The drawing under review shows one solid part. Ordinate dimensions are in mm from its lowest x, y, z. A direction names the side the tool comes from. Give positions to 0.01 mm unless a question says otherwise; leave off trailing zeros. Loops run counter-clockwise (first coordinate to the right, second up) from the corner with the lowest first, then second, coordinate; pieces in that order, holes last. Notation, with made-up numbers: (-8.75, 72) -> (22.25, 72) arc R23 cw to (22.25, 99) -> close; hole circle Ø3 at (-17.75, -3.75). An arc over 180 degrees is marked (long way). Answer in a Markdown table with one row per item. Add a question column.
(1) For pin 1 (21 mm diameter, centred on x = 19, z = 26.5, fed in from +Y); pin 2 (12 mm diameter, centred on x = 29.5, z = 24, fed in from +Y), all flat-tipped, find the tip position at first contact; note any pin that passes through.
(2) For the marked faces 1 and 2, list the 3-axis set-ups (+Z, -Z, +X, -X, +Y, -Y) from which the entire face can be reached by the end or side of a thin tool; tool diameter is ignored.
(3) Consider section C-C on y = 57.5. Write out the cut boundary in (x, z).
(4) Consider section B-B on x = 21. Write out the cut boundary in (y, z).
(5) Consider section D-D on x = 33. Write out the cut boundary in (y, z), then the cut area to 3 significant figures.
(6) Consider section A-A on z = 21. Write out the cut boundary in (x, y), then the cut area to 3 significant figures.
(7) For line 1 (Y direction, x = 12, z = 33); line 2 (X direction, y = 48, z = 22.5), list the stretches that pass through material, from the lowest coordinate up.
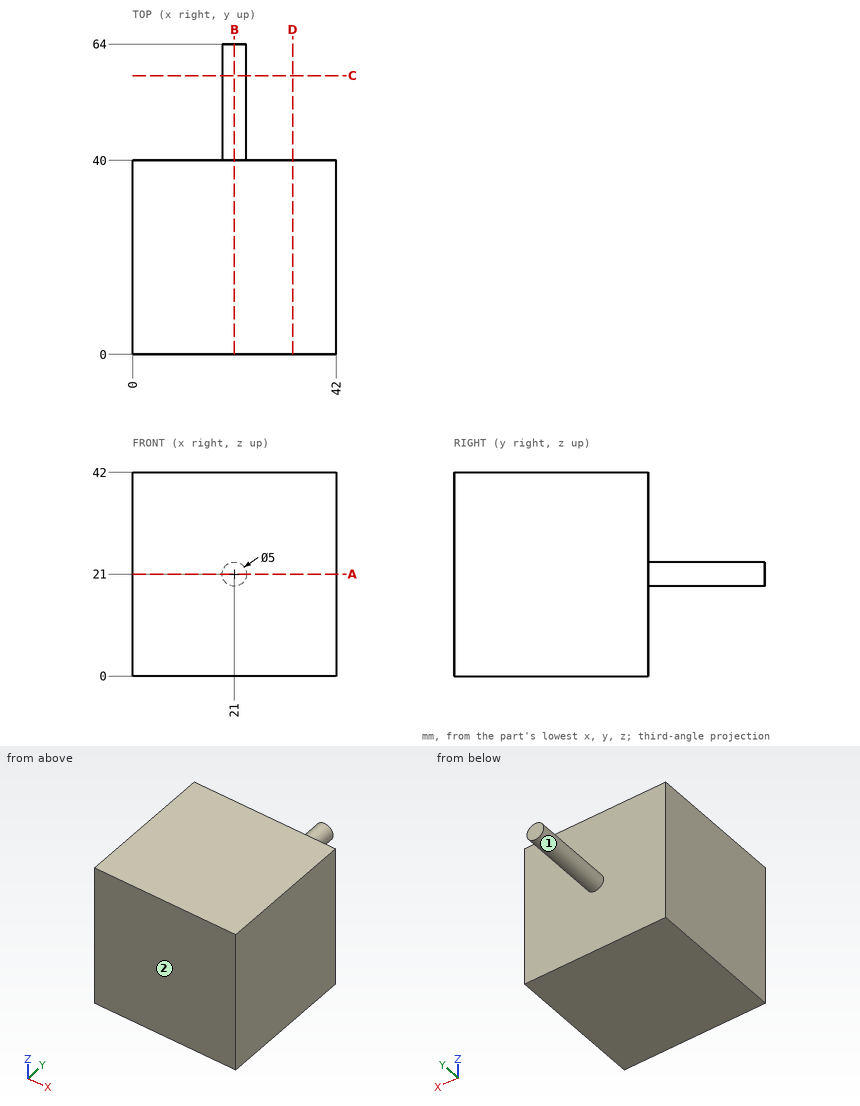
Values follow:
| question | item | result |
|---|---|---|
| 1 | pin 1 | y = 64 |
| 1 | pin 2 | y = 40 |
| 2 | face 1 | +Y |
| 2 | face 2 | +Z, -Z, +X, -X, -Y |
| 3 | outline | circle Ø5 at (21, 21) |
| 4 | outline | (0, 0) -> (40, 0) -> (40, 18.5) -> (64, 18.5) -> (64, 23.5) -> (40, 23.5) -> (40, 42) -> (0, 42) -> close |
| 5 | outline | (0, 0) -> (40, 0) -> (40, 42) -> (0, 42) -> close |
| 5 | area | 1,680 mm2 |
| 6 | outline | (0, 0) -> (42, 0) -> (42, 40) -> (23.5, 40) -> (23.5, 64) -> (18.5, 64) -> (18.5, 40) -> (0, 40) -> close |
| 6 | area | 1,800 mm2 |
| 7 | line 1 | 0 to 40 |
| 7 | line 2 | 19 to 23 |
